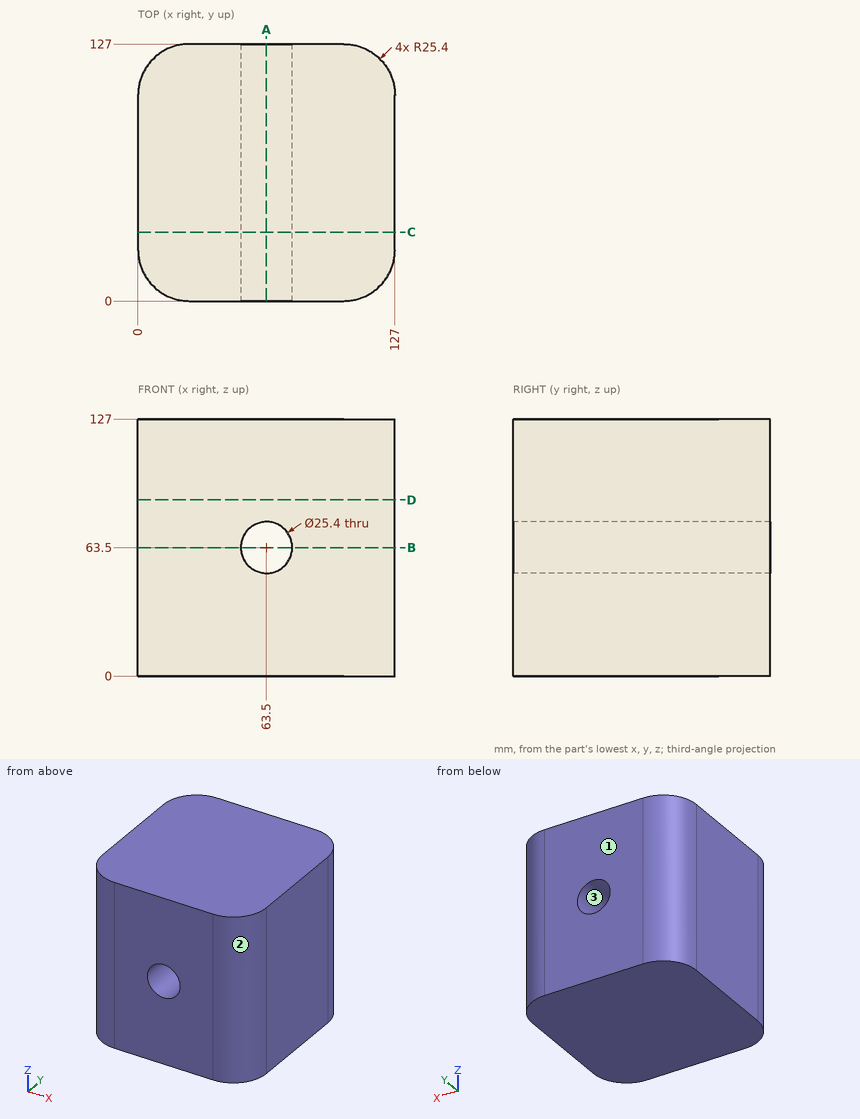
Study the drawing (mm; zero at the part's minimum x, y, z) and answer. Round coordinates to 2 decimals unless told otherwise and drop trailing zeros. Write each loop counter-clockwise with the first axis right and the second up, starting at its lowest first coordinate (ties: lowest second). Pieces come first, ordered by that corner, then holes. Notation, with made-up numbers: (24.25, 67.5) -> (81.25, 67.5) arc R13 ccw to (81.25, 90.5) -> close; hole circle Ø3 at (89, 57). An arc over 180 degrees is marked (long way). Answer as CSV lines item,"result". Start each with the question number.
(1) The part is cut by section C-C, the plane y = 34. Give the vertices of the cut face in (x, z).
(2) The part is cut by section B-B, the plane z = 63.5. Give the vertices of the cut face in (x, y).
(3) The part is cut by section D-D, the plane z = 87. Give the vertices of the cut face in (x, y), then the cut area to 3 significant figures.
(4) The part is cut by section A-A, the plane x = 63.5. Give the vertices of the cut face in (y, z), then the cut area to 3 significant figures.
(5) The mould has two halves that part along X. Classify the marked faces 1, 2 and 3: +X half, -X half, draft (parallel to the pull), parting line (faces both ways), or undercut.
(6) Each of these flat-tipped pins is pushed along its axis until it touches: pin 1 (6 mm diameter, centred on y = 107, z = 32.5, fed in from +X); pin 2 (3 mm diameter, centred on y = 104.5, z = 93.5, fed in from +X); pin 3 (4 mm diameter, centred on y = 20, z = 84, fed in from +X). Where does it stop, or does it pass through?
(7) Find the intervals of material crossed by probe 1 along Z at (x, y) = (63, 82); probe 2 along X at (y, z) = (83.5, 74); probe 3 along Z at (x, y) = (52.5, 51), in increasing order.
Output values:
1,outline,"(0, 0) -> (127, 0) -> (127, 127) -> (0, 127) -> close; hole circle Ø25.4 at (63.5, 63.5)"
2,outline,"(0, 25.4) arc R25.4 ccw to (25.4, 0) -> (50.8, 0) -> (50.8, 127) -> (25.4, 127) arc R25.4 ccw to (0, 101.6) -> close; (76.2, 0) -> (101.6, 0) arc R25.4 ccw to (127, 25.4) -> (127, 101.6) arc R25.4 ccw to (101.6, 127) -> (76.2, 127) -> close"
3,outline,"(0, 25.4) arc R25.4 ccw to (25.4, 0) -> (101.6, 0) arc R25.4 ccw to (127, 25.4) -> (127, 101.6) arc R25.4 ccw to (101.6, 127) -> (25.4, 127) arc R25.4 ccw to (0, 101.6) -> close"
3,area,"15,600 mm²"
4,outline,"(0, 0) -> (127, 0) -> (127, 50.8) -> (0, 50.8) -> close; (0, 76.2) -> (127, 76.2) -> (127, 127) -> (0, 127) -> close"
4,area,"12,900 mm²"
5,face 1,"draft"
5,face 2,"+X half"
5,face 3,"undercut"
6,pin 1,"stops at x = 126.89"
6,pin 2,"stops at x = 126.96"
6,pin 3,"stops at x = 126.77"
7,probe 1,"z = 0 to 50.81, 76.19 to 127"
7,probe 2,"x = 0 to 56.36, 70.64 to 127"
7,probe 3,"z = 0 to 57.15, 69.85 to 127"
